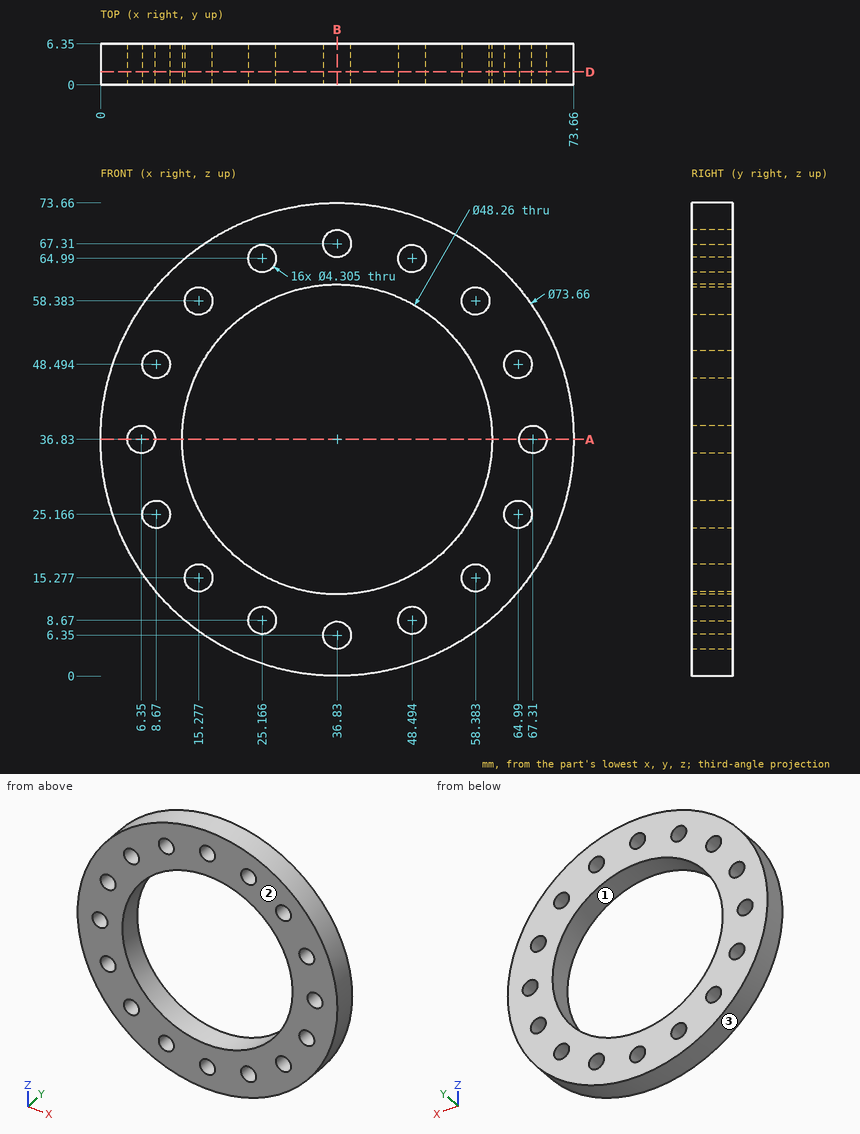
For this review, use the dimensioned drawing (mm, ordinates from the lowest corner) and the shaded views. Round coordinates to 2 decimals unless told otherwise and drop trailing zeros. Write each loop counter-clockwise with the first axis right and the second up, starting at its lowest first coordinate (ties: lowest second). Pieces come first, ordered by that corner, then holes. Notation, with made-up numbers: M 19.25,0.25 L 69.25,0.25 A24 cw 69.25,24.25 Z; hole C 35.25,74 d5. An arc over 180 degrees is marked long. Answer as CSV lines item,"result". Start each with the question number.
Q1. Clearance check with flat-ended pins moving along their axes: P1, Ø3.5, axis at x = 15.28, z = 58.38, coming from the +Y side; P2, Ø3, axis at y = 4, z = 44.5, coming from the +X side; P3, Ø7, axis at x = 48.49, z = 8.67, coming from the -Y side; P4, Ø1.5, axis at x = 15, y = 1, coming from the +Z side. State where each tip first meets the part, or that it passes through.
Q2. Wall thickness on line 1 along Z through (x, y) = (35, 5) (1 decimal); line 2 along X through (y, z) = (1.25, 48.5); line 3 along Z through (x, y) = (48, 3.25) (1 decimal): over which ranges is each line inside the solid? List them lowest first.
Q3. The part is to be moulded in two halves that separate along Z. For the marked faces 1, 2 and 3, say which applies: +Z half, -Z half, draft (parallel to the pull), parting line (faces both ways), or undercut.
Q4. Consider section A-A, the plane z = 36.83. Give the boundary of the cut face in (x, y), then the cut area to 3 significant figures.
Q5. Consider section D-D, the plane y = 2. State how many separate pieces and enclosed holes the cut face has, then the cut area to 3 significant figures.
Q6. Consider section B-B, the plane x = 36.83. Give the boundary of the cut face in (y, z), then the cut area to 3 significant figures.
Result set:
1,P1,"passes through"
1,P2,"stops at x = 73.14"
1,P3,"stops at y = 0"
1,P4,"stops at z = 67.03"
2,line 1,"z = 0 to 5.2, 7.5 to 12.8, 60.9 to 66.2, 68.4 to 73.6"
2,line 2,"x = 1.9 to 6.52, 10.82 to 15.71, 57.95 to 62.84, 67.14 to 71.76"
2,line 3,"z = 1.7 to 6.6, 10.8 to 15.4, 58.2 to 62.9, 67.1 to 71.9"
3,face 1,"undercut"
3,face 2,"draft"
3,face 3,"parting line"
4,outline,"M 0,0 L 4.2,0 L 4.2,6.35 L 0,6.35 Z; M 8.5,0 L 12.7,0 L 12.7,6.35 L 8.5,6.35 Z; M 60.96,0 L 65.16,0 L 65.16,6.35 L 60.96,6.35 Z; M 69.46,0 L 73.66,0 L 73.66,6.35 L 69.46,6.35 Z"
4,area,"107 mm²"
5,separate pieces,"1"
5,enclosed holes,"17"
5,area,"2,200 mm²"
6,outline,"M 0,0 L 6.35,0 L 6.35,4.2 L 0,4.2 Z; M 0,8.5 L 6.35,8.5 L 6.35,12.7 L 0,12.7 Z; M 0,60.96 L 6.35,60.96 L 6.35,65.16 L 0,65.16 Z; M 0,69.46 L 6.35,69.46 L 6.35,73.66 L 0,73.66 Z"
6,area,"107 mm²"
